The listing builds one solid part. Answer for the finished solid, in the listing's coordinates (mm). A direction names the side the tool comes from. Round coordinates to 2 decimals unless told otherwise and drop trailing zeros. Write each loop counter-clockwise with the first axis right and the second up, starting at its lowest first coordinate (ties: lowest second). Pieces come first, ordered by that corner, then holes. Notation, with made-up numbers: (62.5, -6.75) - (102.5, -6.75) arc R23 ccw to (102.5, 6.25) - close; hole circle Ø8 at (-17.75, 12). An arc over 180 degrees is marked (long way). Answer in a Markdown table with one row per item.
from build123d import *

# Parameters (mm, degrees)
CYLINDER005_R     = 1.4
CYLINDER005_DEPTH = 10
SKETCH001_W       = 28.4
SKETCH001_H       = 68.4
SKETCH001_W_2     = 25.4
SKETCH001_H_2     = 65.4
EXTRUDE001_DEPTH  = 4
SKETCH_W          = 28.4
SKETCH_H          = 68.4
SKETCH_R          = 1.4
SKETCH_W_2        = 22
SKETCH_H_2        = 43
EXTRUDE_DEPTH     = 1


with BuildPart() as cylinder005:
    # Cylinder005 → Cylinder005 (new body)
    with BuildSketch(Plane(origin=(-5, 2.5, -5), x_dir=(1, 0, 0), z_dir=(0, 0, 1))):
        Circle(CYLINDER005_R)
    extrude(amount=CYLINDER005_DEPTH)


with BuildPart() as extrude001:
    # Sketch001 → Extrude001 (new body)
    with BuildSketch(Plane.XY.offset(1)):
        with Locations((0, -21.5)):
            Rectangle(SKETCH001_W, SKETCH001_H)
        with Locations((0, -21.5)):
            Rectangle(SKETCH001_W_2, SKETCH001_H_2, mode=Mode.SUBTRACT)
    extrude(amount=-EXTRUDE001_DEPTH)


with BuildPart() as body001:
    # Sketch → Extrude (new body)
    with BuildSketch(Plane.XY.offset(1)):
        with Locations((0, -21.5)):
            Rectangle(SKETCH_W, SKETCH_H)
        with Locations((-5, 2.5)):
            Circle(SKETCH_R, mode=Mode.SUBTRACT)
        with Locations((5, 2.5)):
            Circle(SKETCH_R, mode=Mode.SUBTRACT)
        with Locations((-5, -45.5)):
            Circle(SKETCH_R, mode=Mode.SUBTRACT)
        with Locations((5, -45.5)):
            Circle(SKETCH_R, mode=Mode.SUBTRACT)
        with Locations((0, -21.5)):
            Rectangle(SKETCH_W_2, SKETCH_H_2, mode=Mode.SUBTRACT)
    extrude(amount=EXTRUDE_DEPTH)

    # Fusion012: union Extrude001
    add(extrude001.part)

    # Cut001: cut Cylinder005
    add(cylinder005.part, mode=Mode.SUBTRACT)


with BuildPart() as body003:
    # Part__Mirroring002: instance of Body001
    add(body001.part.mirror(Plane(origin=(0, -21.5, 0), x_dir=(1, 0, 0), z_dir=(0, 1, 0))))


with BuildPart() as part_mirroring004:
    # Part__Mirroring004: instance of Body003
    add(body003.part.mirror(Plane(origin=(0, -21.5, 0), x_dir=(0, -1, 0), z_dir=(1, 0, 0))))


solid = part_mirroring004.part
(1) Flat-ended cylindrical pins translate along their axes: pin 1 (2 mm diameter, centred on x = 5, y = -45.5, fed in from -Z); pin 2 (4 mm diameter, centred on x = 1.5, y = -1.5, fed in from -Z). Find the tip coordinate at first contact, or state that the pin passes through.
Checked values:
| item | result |
|---|---|
| pin 1 | passes through |
| pin 2 | stops at z = 1 |
(2) Section A-A (x = -9.75) is taken. Give the vertices of the cut face in (y, z).
Checked values:
| item | result |
|---|---|
| outline | (-55.7, -3) - (-54.2, -3) - (-54.2, 1) - (-43, 1) - (-43, 2) - (-55.7, 2) - close; (0, 1) - (11.2, 1) - (11.2, -3) - (12.7, -3) - (12.7, 2) - (0, 2) - close |
(3) Find the intervals of material crossed by line 1 (Y direction, x = 5, z = 1.4); line 2 (X direction, y = 2.5, z = 1.55); line 3 (X direction, y = -33, z = -0.1), in increasing order.
Checked values:
| item | result |
|---|---|
| line 1 | y = -55.7 to -46.9, -44.1 to -43, 0 to 1.1, 3.9 to 12.7 |
| line 2 | x = -14.2 to -6.4, -3.6 to 3.6, 6.4 to 14.2 |
| line 3 | x = -14.2 to -12.7, 12.7 to 14.2 |
(4) For a pull along Y with two mould halves and no side action, classify faces 3 (the flat face through (11.5, -29.2, 1)), 4 (the flat face through (14, -22, -3)), 5 (the flat face through (0, 12.7, 0)), 6 (the cylindrical face through (3.665, 2.079, 1.493)) as pulls with the +Y half, pulls with the -Y half, needs draft (parallel to the pull), parting line crosses it, or undercut.
Checked values:
| item | result |
|---|---|
| face 3 | undercut |
| face 4 | needs draft |
| face 5 | pulls with the +Y half |
| face 6 | undercut |
(5) Section D-D (z = -1.25) is taken. Give the vertices of the cut face in (x, y), and give its area (3 significant figures).
Checked values:
| item | result |
|---|---|
| outline | (-14.2, -55.7) - (14.2, -55.7) - (14.2, 12.7) - (-14.2, 12.7) - close; hole (-12.7, -54.2) - (12.7, -54.2) - (12.7, 11.2) - (-12.7, 11.2) - close |
| area | 281 mm2 |
(6) Section B-B (x = 5) is taken. Give the vertices of the cut face in (y, z), and give its area (3 significant figures).
Checked values:
| item | result |
|---|---|
| outline | (-55.7, -3) - (-54.2, -3) - (-54.2, 1) - (-46.9, 1) - (-46.9, 2) - (-55.7, 2) - close; (-44.1, 1) - (-43, 1) - (-43, 2) - (-44.1, 2) - close; (0, 1) - (1.1, 1) - (1.1, 2) - (0, 2) - close; (3.9, 1) - (11.2, 1) - (11.2, -3) - (12.7, -3) - (12.7, 2) - (3.9, 2) - close |
| area | 31.8 mm2 |
(7) For faces 1 (the flat face through (0, -54.2, -1)), 2 (the flat face through (0, -55.7, 0)), determine the directions among +Z, -Z, +X, -X, +Y, -Y from which every point of the face is accessible in a straight line to the end or side of a thin tool.
Checked values:
| item | result |
|---|---|
| face 1 | -Z |
| face 2 | +Z, -Z, +X, -X, -Y |
(8) Section C-C (y = 2.5) is taken. Give the vertices of the cut face in (x, z), and give its area (3 significant figures).
Checked values:
| item | result |
|---|---|
| outline | (-14.2, -3) - (-12.7, -3) - (-12.7, 1) - (-6.4, 1) - (-6.4, 2) - (-14.2, 2) - close; (-3.6, 1) - (3.6, 1) - (3.6, 2) - (-3.6, 2) - close; (6.4, 1) - (12.7, 1) - (12.7, -3) - (14.2, -3) - (14.2, 2) - (6.4, 2) - close |
| area | 34.8 mm2 |
